Autodesk Fusion 360 part; units mm, degrees
sketch "Sketch1" plane through (0, 0, 0) normal (0, 1, 0) x (1, 0, 0)
  line L0 (0, 0) -> (45, 0)
  line L1 (45, 0) -> (45, -60)
  line L2 (45, -60) -> (0, -60)
  line L3 (0, -60) -> (0, 0)
  dimension "d9" = 45
  dimension "d10" = 60
extrude "Extrude1" add sketch "Sketch1" against normal blind 8
sketch "Sketch3" plane through (0, 0, 0) normal (0, 1, 0) x (-1, 0, 0)
  line L0 (0, 60) -> (-45, 60)
  line L1 (-45, 60) -> (-45, 0)
  line L2 (-45, 0) -> (0, 0)
  line L3 (0, 0) -> (0, 60)
  line L4 (-45, 60) -> (0, 60)
  line L5 (0, 60) -> (0, 52)
  line L6 (0, 52) -> (-45, 52)
  line L7 (-45, 52) -> (-45, 60)
  dimension "d13" = 45
  dimension "d14" = 8
extrude "Extrude2" add sketch "Sketch3" along normal blind 18 contours L0 L1 L3 L4 L5 L6 L7
sketch "Sketch4" plane through (0, 0, 52) normal (0, 0, -1) x (1, 0, 0)
  line L0 (45, 0) -> (0, 0)
  line L1 (0, 0) -> (0, -18)
  line L2 (0, -18) -> (45, -18)
  line L3 (45, -18) -> (45, 0)
  line L4 (0, -18) -> (45, -18)
  line L5 (45, -18) -> (45, -10)
  line L6 (45, -10) -> (0, -10)
  line L7 (0, -10) -> (0, -18)
  dimension "d17" = 45
  dimension "d18" = 8
extrude "Extrude3" add sketch "Sketch4" along normal blind 52 contours L1 L2 L3 L4 L5 L6 L7
sketch "Sketch5" plane through (0, -8, 0) normal (0, -1, 0) x (1, 0, 0)
  line L0 (45, 60) -> (0, 60)
  line L1 (0, 60) -> (0, 0)
  line L2 (0, 0) -> (45, 0)
  line L3 (45, 0) -> (45, 60)
  line L4 (0, 0) -> (45, 0)
  line L5 (45, 0) -> (45, 8)
  line L6 (45, 8) -> (0, 8)
  line L7 (0, 8) -> (0, 0)
  dimension "d21" = 45
  dimension "d22" = 8
extrude "Extrude4" add sketch "Sketch5" along normal blind 20 contours L1 L2 L3 L4 L5 L6 L7
sketch "Sketch6" plane through (0, 0, 8) normal (0, 0, 1) x (-1, 0, 0)
  line L0 (-45, 8) -> (0, 8)
  line L1 (0, 8) -> (0, 28)
  line L2 (0, 28) -> (-45, 28)
  line L3 (-45, 28) -> (-45, 8)
  line L4 (-22.5, 28) -> (-30, 28)
  line L5 (-22.5, 28) -> (-15, 28)
  line L6 (-30, 28) -> (-45, 8)
  line L7 (-15, 28) -> (0, 8)
  dimension "d25" = 7.5
  dimension "d26" = 7.5
extrude "Extrude5" cut sketch "Sketch6" against normal blind 8 contours L2 L3 L6 | L1 L2 L7
sketch "Sketch7" plane through (0, 0, 8) normal (0, 0, 1) x (-1, 0, 0)
  line L0 (0, 8) -> (-15, 28)
  line L1 (-15, 28) -> (-30, 28)
  line L2 (-30, 28) -> (-45, 8)
  line L3 (-45, 8) -> (0, 8)
  line L4 (-15, 28) -> (-30, 28)
  line L5 (-30, 28) -> (-33.75, 23)
  line L6 (-33.75, 23) -> (-11.25, 23)
  line L7 (-11.25, 23) -> (-15, 28)
  dimension "d29" = 15
  dimension "d30" = 5
extrude "Extrude6" add sketch "Sketch7" along normal blind 10 contours L0 L1 L2 L4 L5 L6 L7
sketch "Sketch8" plane through (0, 18, 0) normal (0, 1, 0) x (-1, 0, 0)
  line L0 (0, 0) -> (0, 60)
  line L1 (0, 60) -> (-45, 60)
  line L2 (-45, 60) -> (-45, 0)
  line L3 (-45, 0) -> (0, 0)
  line L4 (-45, 0) -> (0, 0)
  line L5 (0, 0) -> (0, 8)
  line L6 (0, 8) -> (-45, 8)
  line L7 (-45, 8) -> (-45, 0)
  dimension "d33" = 45
  dimension "d34" = 8
extrude "Extrude7" add sketch "Sketch8" along normal blind 20 contours L0 L2 L3 L4 L5 L6 L7
sketch "Sketch9" plane through (0, 0, 8) normal (0, 0, 1) x (-1, 0, 0)
  line L0 (0, -18) -> (-45, -18)
  line L1 (-45, -18) -> (-45, -38)
  line L2 (-45, -38) -> (0, -38)
  line L3 (0, -38) -> (0, -18)
  line L4 (-22.5, -38) -> (-30, -38)
  line L5 (-22.5, -38) -> (-15, -38)
  line L6 (-15, -38) -> (0, -18)
  line L7 (-30, -38) -> (-45, -18)
  dimension "d37" = 7.5
  dimension "d38" = 7.5
extrude "Extrude8" cut sketch "Sketch9" against normal blind 8 contours L2 L3 L6 | L1 L2 L7
sketch "Sketch10" plane through (0, 0, 8) normal (0, 0, 1) x (-1, 0, 0)
  line L0 (-15, -38) -> (0, -18)
  line L1 (0, -18) -> (-45, -18)
  line L2 (-45, -18) -> (-30, -38)
  line L3 (-30, -38) -> (-15, -38)
  line L4 (-15, -38) -> (-11.25, -33)
  line L5 (-15, -38) -> (-30, -38)
  line L6 (-30, -38) -> (-33.75, -33)
  line L7 (-11.25, -33) -> (-33.75, -33)
  dimension "d41" = 5
extrude "Extrude9" add sketch "Sketch10" along normal blind 10 contours L0 L2 L3 L4 L5 L6 L7
equation "haed = 60 mm"
equation "pinni_breidd = 15 mm"
equation "thykkt = 8 mm"
equation "haed_pinni = 10 mm"
equation "flotur = 20 mm"
equation "breidd = 3 * pinni_breidd"
equation "bil = 10 mm"
equation "pinni_lengd = 5 mm"
equation "d9 = breidd"
equation "d10 = haed"
equation "d13 = breidd"
equation "d14 = thykkt"
equation "d15 = bil + thykkt"
equation "d17 = breidd"
equation "d18 = thykkt"
equation "d19 = haed - thykkt"
equation "d21 = breidd"
equation "d22 = thykkt"
equation "d23 = flotur"
equation "d25 = pinni_breidd / 2"
equation "d26 = pinni_breidd / 2"
equation "d30 = pinni_lengd"
equation "d31 = haed_pinni"
equation "d33 = breidd"
equation "d34 = thykkt"
equation "d35 = flotur"
equation "d37 = pinni_breidd / 2"
equation "d38 = pinni_breidd / 2"
equation "d41 = pinni_lengd"
equation "d42 = haed_pinni"
Geometry: final body of the model. Coordinates: model frame, mm. A direction names the side the tool comes from. Round coordinates to 2 decimals unless told otherwise and drop trailing zeros. Loops run counter-clockwise (first coordinate to the right, second up) from the corner with the lowest first, then second, coordinate; pieces in that order, holes last. Notation, with made-up numbers: (34.5, -2) - (56.5, -2) arc R11 ccw to (56.5, 6) - close; hole circle Ø11 at (9, 77). An arc over 180 degrees is marked (long way). Write each question's results on one line, items separated by ' | '. Start each with the question number.
1) Cut plane B-B on x = 4.5. Return loops of the section in (y, z), then the cut area to 3 significant figures.
2) Mould query, pull axis Y, two halves, no side actions, for faces 1 (the face through (23, 35, 18)), 2 (the face through (22, 5, 52)), 3 (the face through (22, -28, 9)), 4 (the face through (22, 33, 13)). Classes: released by +Y, released by -Y, zero draft, split by the parting line, or undercut.
3) First-contact query: P1, Ø5, axis at y = 19.5, z = 41.5, coming from the +X side; P2, Ø2, axis at x = 31, y = -13.5, coming from the +Z side; P3, Ø5.5, axis at x = 26, y = 35, coming from the +Z side; P4, Ø5, axis at x = 16, z = 41, coming from the -Y side. Flat tips, straight axial feed; report the tip coordinate or a pass-through.
4) Access query for faces 5 (the face through (22, 18, 34)), 6 (the face through (9, 30, 5)), 7 (the face through (22, 0, 26)). Directions: +Z, -Z, +X, -X, +Y, -Y. A direction counts if a zero-diameter tool reaches every point of the face in a straight line with its end or side. Return the directions, or none.
5) Line query: probe 1 along Y at (x, z) = (9.5, 45.5); probe 2 along Y at (x, z) = (14.5, 12.5); probe 3 along Y at (x, z) = (17, 4). Output: solid intervals per line, ascending. Write a range as [from, to].
6) Cut plane D-D on y = -21. Return loops of the section in (x, z).
7) Cut plane A-A on z = 6.5. Return loops of the section in (x, y).
8) Cut plane C-C on z = 49.5. Return loops of the section in (x, y).
Verdict:
1) outline: (-14, 0) - (0, 0) - (0, 52) - (10, 52) - (10, 0) - (24, 0) - (24, 8) - (18, 8) - (18, 60) - (-8, 60) - (-8, 8) - (-14, 8) - close | area: 1,140 mm2
2) face 1: zero draft | face 2: undercut | face 3: released by -Y | face 4: undercut
3) P1: stops at x = 45 | P2: stops at z = 8 | P3: stops at z = 18 | P4: stops at y = -8
4) face 5: +Z, +X, -X | face 6: +Z, -Z, -X, +Y | face 7: -Z, +X, -X
5) probe 1: y = [-8, 0], [10, 18] | probe 2: y = [-27.33, -23], [-8, 0], [10, 18], [33, 37.33] | probe 3: y = [-28, 0], [10, 38]
6) outline: (9.75, 0) - (35.25, 0) - (35.25, 8) - (9.75, 8) - close
7) outline: (0, -8) - (15, -28) - (30, -28) - (45, -8) - (45, 0) - (0, 0) - close; (0, 10) - (45, 10) - (45, 18) - (30, 38) - (15, 38) - (0, 18) - close
8) outline: (0, -8) - (45, -8) - (45, 0) - (0, 0) - close; (0, 10) - (45, 10) - (45, 18) - (0, 18) - close
